Source: CAD feature listing. Evaluate the final solid. Frame: model axes, mm. Round coordinates to 2 decimals unless told otherwise and drop trailing zeros. Loops run counter-clockwise (first coordinate to the right, second up) from the corner with the lowest first, then second, coordinate; pieces in that order, holes last. Notation, with made-up numbers: (79, -21) - (109, -21) arc R26 cw to (109, 17) - close; hole circle Ø2 at (-22.75, 8.5). An arc over 180 degrees is marked (long way). One line per question, with ' | ' between items. Start each with the question number.
1. Cut plane B-B (y = 543). Return loops of the section in (x, z).
2. Ray query, line 1 (X direction, y = 91, z = 53.5); line 2 (Z direction, x = 334.5, y = -261); line 3 (X direction, y = -177, z = -641). Return the intervals inside material, ascending.
3. Pin query (flat end, axial travel): pin 1 (8 mm diameter, centred on x = -335, z = -641.5, fed in from +Y); pin 2 (1 mm diameter, centred on x = 600.5, z = -622, fed in from -Y). Return the tip coordinate at first contact, or that it passes through.
4. Cut plane C-C (x = -401). Return loops of the section in (y, z).
5. Cut plane A-A (z = 39). Return loops of the section in (x, y), then the cut area to 3 significant figures.
6. Cut plane D-D (z = -352). Return loops of the section in (x, y).
```python
from build123d import *

# Parameters (mm, degrees)
F0_W     = 2000
F0_H     = 1000
F1_DEPTH = 100
F2_W     = 600
F2_H     = 425
F3_DEPTH = 640
F4_W     = 100
F4_H     = 50
F5_DEPTH = 1000
F6_W     = 100
F6_H     = 50
F7_DEPTH = 1000
F8_W     = 100
F8_H     = 50
F9_DEPTH = 2000


with BuildPart() as f1:
    # F0 (on Top) → F1 (new body)
    with BuildSketch(Plane.XY):
        with Locations((10.600965, 127.579693)):
            Rectangle(F0_W, F0_H)
    extrude(amount=F1_DEPTH)

    # F2 (on face) → F3 (cut)
    with BuildSketch(Plane.XY.offset(100)):
        with Locations((-639.399035, 365.079693)):
            Rectangle(F2_W, F2_H)
        with Locations((-639.399035, -109.920307)):
            Rectangle(F2_W, F2_H)
        with Locations((10.600965, 365.079693)):
            Rectangle(F2_W, F2_H)
        with Locations((660.600965, 365.079693)):
            Rectangle(F2_W, F2_H)
        with Locations((10.600965, -109.920307)):
            Rectangle(F2_W, F2_H)
        with Locations((660.600965, -109.920307)):
            Rectangle(F2_W, F2_H)
    extrude(amount=-F3_DEPTH, mode=Mode.SUBTRACT)

    # F4 (on face) → F5 (join)
    with BuildSketch(Plane.XY.offset(100)):
        with Locations((960.600965, 602.579693)):
            Rectangle(F4_W, F4_H)
        with Locations((-939.399035, -347.420307)):
            Rectangle(F4_W, F4_H)
        with Locations((-939.399035, 602.579693)):
            Rectangle(F4_W, F4_H)
        with Locations((960.600965, -347.420307)):
            Rectangle(F4_W, F4_H)
    extrude(amount=-F5_DEPTH)

    # F6 (on face) → F7 (join)
    with BuildSketch(Plane.XZ.offset(372.420307)):
        with Locations((-939.399035, -625)):
            Rectangle(F6_W, F6_H)
        with Locations((960.600965, -625)):
            Rectangle(F6_W, F6_H)
    extrude(amount=-F7_DEPTH)

    # F8 (on face) → F9 (join)
    with BuildSketch(Plane.YZ.offset(1010.600965)):
        with Locations((127.579693, -625)):
            Rectangle(F8_W, F8_H)
    extrude(amount=-F9_DEPTH)


solid = f1.part
```
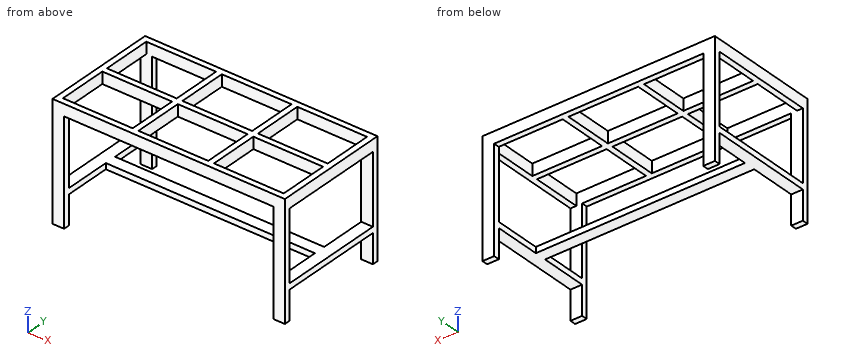
Answers follow:
1) outline: (-989.4, -650) - (-889.4, -650) - (-889.4, -600) - (-989.4, -600) - close; (-989.4, 0) - (-939.4, 0) - (-939.4, 100) - (-989.4, 100) - close; (-339.4, 0) - (-289.4, 0) - (-289.4, 100) - (-339.4, 100) - close; (310.6, 0) - (360.6, 0) - (360.6, 100) - (310.6, 100) - close; (910.6, -650) - (1010.6, -650) - (1010.6, -600) - (910.6, -600) - close; (960.6, 0) - (1010.6, 0) - (1010.6, 100) - (960.6, 100) - close
2) line 1: x = -989.4 to -939.4, -339.4 to -289.4, 310.6 to 360.6, 960.6 to 1010.6 | line 2: z = 0 to 100 | line 3: x = -989.4 to -889.4, 910.6 to 1010.6
3) pin 1: stops at y = 177.58 | pin 2: stops at y = 77.58
4) outline: (-372.42, 0) - (-322.42, 0) - (-322.42, 100) - (-372.42, 100) - close; (77.58, -650) - (177.58, -650) - (177.58, -600) - (77.58, -600) - close; (102.58, 0) - (152.58, 0) - (152.58, 100) - (102.58, 100) - close; (577.58, 0) - (627.58, 0) - (627.58, 100) - (577.58, 100) - close
5) outline: (-989.4, -372.42) - (1010.6, -372.42) - (1010.6, 627.58) - (-989.4, 627.58) - close; hole (-939.4, -322.42) - (-339.4, -322.42) - (-339.4, 102.58) - (-939.4, 102.58) - close; hole (-939.4, 152.58) - (-339.4, 152.58) - (-339.4, 577.58) - (-939.4, 577.58) - close; hole (-289.4, -322.42) - (310.6, -322.42) - (310.6, 102.58) - (-289.4, 102.58) - close; hole (-289.4, 152.58) - (310.6, 152.58) - (310.6, 577.58) - (-289.4, 577.58) - close; hole (360.6, -322.42) - (960.6, -322.42) - (960.6, 102.58) - (360.6, 102.58) - close; hole (360.6, 152.58) - (960.6, 152.58) - (960.6, 577.58) - (360.6, 577.58) - close | area: 470,000 mm2
6) outline: (-989.4, -372.42) - (-889.4, -372.42) - (-889.4, -322.42) - (-989.4, -322.42) - close; (-989.4, 577.58) - (-889.4, 577.58) - (-889.4, 627.58) - (-989.4, 627.58) - close; (910.6, -372.42) - (1010.6, -372.42) - (1010.6, -322.42) - (910.6, -322.42) - close; (910.6, 577.58) - (1010.6, 577.58) - (1010.6, 627.58) - (910.6, 627.58) - close
